Source: CAD feature listing. Evaluate the final solid. Frame: model axes, mm. Face numbers are marked on the shaded views. A direction names the side the tool comes from. Round coordinates to 2 decimals unless told otherwise and drop trailing zeros. Loops run counter-clockwise (first coordinate to the right, second up) from the corner with the lowest first, then second, coordinate; pieces in that order, holes last.
(1) Section C-C, the plane x = -12.75. Return the cut outline in (y, z).
(2) Section A-A, the plane z = 31.75. Return the cut outline in (x, y) (3 decimals), plus the area to 3 significant figures.
(3) Section B-B, the plane x = -5.5. Return the cut outline in (y, z), plus the area to 3 significant figures.
(4) First-contact query: pin 1 Ø3 at (x, z) = (-4.5, 30.5) entering from -Y; pin 2 Ø8 at (x, y) = (-8.5, -33) entering from -Z; pin 3 Ø5 at (x, z) = (-11.07, 31.75) entering from +Y; pin 4 Ø5 at (y, z) = (-26, 12.5) entering from +X. Flat tips, straight axial feed; report the tip coordinate or a pass-through.
(5) Mould query, pull axis X, two halves, no side actions, for the marked faces 4, 5 and 6. Classes: pulls with the +X half, pulls with the -X half, needs draft (parallel to the pull), parting line crosses it, or undercut.
(6) Set-up query: the marked faces 1, 2 and 3. Return all of +Z, -Z, +X, -X, +Y, -Y with unobstructed straight access to the full face (end or side cutting, diameter ignored); none if empty.
(7) Material intervals for probe 1 along Z at (x, y) = (-21, -30); probe 2 along Y at (x, z) = (-12.25, 28); probe 3 along X at (y, z) = (-30.5, 13.5) (3 decimals), sorted ascending.
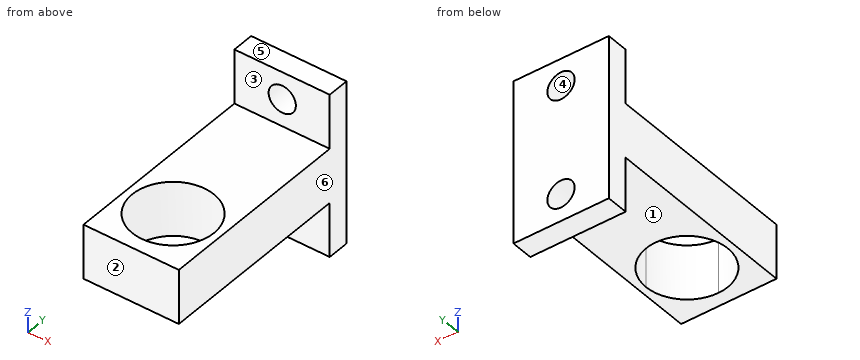
```python
from build123d import *

# Parameters (mm, degrees)
F1_DEPTH = 50.8
F2_W     = 22.225
F2_H     = 12.7
F3_DEPTH = 45.72
F5_DEPTH = 25.401


with BuildPart() as f1:
    # F0 (on Front) → F1 (new body)
    with BuildSketch(Plane.XZ):
        with BuildLine():
            ThreePointArc((-7.8994, 31.75), (-11.0744, 34.925), (-14.2494, 31.75))
            ThreePointArc((-14.2494, 31.75), (-11.0744, 28.575), (-7.8994, 31.75))
        make_face()
        with BuildLine():
            ThreePointArc((-7.8994, 6.35), (-11.0744, 9.525), (-14.2494, 6.35))
            ThreePointArc((-14.2494, 6.35), (-11.0744, 3.175), (-7.8994, 6.35))
        make_face()
        Polygon((-22.225, 0), (0, 0), (0, 38.1), (-22.225, 38.1), (-22.225, 31.75), (-22.225, 25.4), (-22.225, 12.7), (-22.225, 6.35), align=None)
        with BuildLine():
            ThreePointArc((-7.8994, 6.35), (-11.0744, 3.175), (-14.2494, 6.35))
            ThreePointArc((-14.2494, 6.35), (-11.0744, 9.525), (-7.8994, 6.35))
        make_face(mode=Mode.SUBTRACT)
        with BuildLine():
            ThreePointArc((-7.8994, 31.75), (-11.0744, 28.575), (-14.2494, 31.75))
            ThreePointArc((-14.2494, 31.75), (-11.0744, 34.925), (-7.8994, 31.75))
        make_face(mode=Mode.SUBTRACT)
    extrude(amount=F1_DEPTH)

    # F2 (on face) → F3 (cut)
    with BuildSketch(Plane.XZ.offset(50.8)):
        with Locations((-11.1125, 31.75)):
            Rectangle(F2_W, F2_H)
        with Locations((-11.1125, 6.35)):
            Rectangle(F2_W, F2_H)
    extrude(amount=-F3_DEPTH, mode=Mode.SUBTRACT)

    # F4 (on face) → F5 (cut, through all)
    with BuildSketch(Plane.XY.offset(25.4)):
        with BuildLine():
            ThreePointArc((-11.1125, -47.625), (-4.377308, -44.835192), (-1.5875, -38.1))
            ThreePointArc((-1.5875, -38.1), (-17.847692, -31.364808), (-11.1125, -47.625))
        make_face()
    extrude(amount=-F5_DEPTH, mode=Mode.SUBTRACT)


solid = f1.part
```
Output values:
1. outline: (-50.8, 12.7) - (-47.48, 12.7) - (-47.48, 25.4) - (-50.8, 25.4) - close; (-28.72, 12.7) - (-5.08, 12.7) - (-5.08, 9.05) - (0, 9.05) - (0, 29.05) - (-5.08, 29.05) - (-5.08, 25.4) - (-28.72, 25.4) - close; (-5.08, 0) - (0, 0) - (0, 3.65) - (-5.08, 3.65) - close; (-5.08, 34.45) - (0, 34.45) - (0, 38.1) - (-5.08, 38.1) - close
2. outline: (-22.225, -5.08) - (-14.249, -5.08) - (-14.249, 0) - (-22.225, 0) - close; (-7.899, -5.08) - (0, -5.08) - (0, 0) - (-7.899, 0) - close
2. area: 80.6 mm2
3. outline: (-50.8, 12.7) - (-45.8, 12.7) - (-45.8, 25.4) - (-50.8, 25.4) - close; (-30.4, 12.7) - (-5.08, 12.7) - (-5.08, 0) - (0, 0) - (0, 38.1) - (-5.08, 38.1) - (-5.08, 25.4) - (-30.4, 25.4) - close
3. area: 579 mm2
4. pin 1: stops at y = -5.08
4. pin 2: stops at z = 12.7
4. pin 3: passes through
4. pin 4: stops at x = 0
5. face 4: undercut
5. face 5: needs draft
5. face 6: pulls with the +X half
6. face 1: -Z, +X, -X, -Y
6. face 2: +Z, -Z, +X, -X, -Y
6. face 3: +Z, +X, -X, -Y
7. probe 1: z = 12.7 to 25.4
7. probe 2: y = -5.08 to 0
7. probe 3: x = -22.225 to -16.854, -5.371 to 0
